For this review, take the finished solid that the model builds, in its own axes (mm). Face numbers are marked on the shaded views. A direction names the side the tool comes from. Coordinates: 2 decimals unless noted, no trailing zeros. Order: outer loops, then holes, each group sorted by start corner. A loop starts at its lowest first (then second) coordinate and runs counter-clockwise, first axis right, second up. Notation, with made-up numbers: M -34.5,36.5 L 3.5,36.5 A13 cw 3.5,44.5 Z; hole C 26.25,-34 d1. An arc over 180 degrees is marked long. Use CSV: the item, a comma, the result in double quotes.
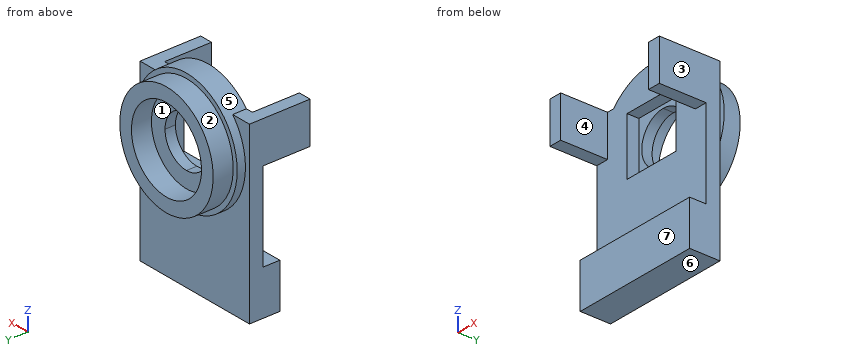
```python
from build123d import *

# Parameters (mm, degrees)
SKETCH2_W           = 8.34
SKETCH2_H           = 8.34
BOSS_EXTRUDE2_DEPTH = 1.5
CUT_EXTRUDE1_DEPTH  = 1.5
BOSS_EXTRUDE4_DEPTH = 3.2
SKETCH6_R           = 8.685
SKETCH6_W           = 11.34
SKETCH6_H           = 11.34
BOSS_EXTRUDE5_DEPTH = 3.2
SKETCH8_R           = 8
SKETCH8_R_2         = 6
BOSS_EXTRUDE6_DEPTH = 2.9
BOSS_EXTRUDE7_START = -2
BOSS_EXTRUDE7_DEPTH = 2
SKETCH11_W          = 18.74
SKETCH11_H          = 6.5
BOSS_EXTRUDE8_DEPTH = 2.4
SKETCH12_W          = 1.85
SKETCH12_H          = 6
BOSS_EXTRUDE9_DEPTH = 6.8


with BuildPart() as part:
    # Sketch2 → Boss-Extrude2 (new body)
    with BuildSketch(Plane(origin=(0, 0, 0), x_dir=(1, 0, 0), z_dir=(0, 1, 0))):
        with Locations((2.034857004, -1.978756257)):
            Rectangle(SKETCH2_W, SKETCH2_H)
    extrude(amount=BOSS_EXTRUDE2_DEPTH)

    # Sketch3 → Cut-Extrude1 (cut)
    with BuildSketch(Plane(origin=(0, 1.5, 0), x_dir=(1, 0, 0), z_dir=(0, 1, 0))):
        with BuildLine():
            ThreePointArc((5.704857004, -1.978756257), (4.629938891, 0.61632563), (2.034857004, 1.691243743))
            Line((2.034857004, 1.691243743), (2.034857004, -5.648756257))
            ThreePointArc((2.034857004, -5.648756257), (4.629938891, -4.573838143), (5.704857004, -1.978756257))
        make_face()
        with BuildLine():
            Line((2.034857004, -5.648756257), (2.034857004, 1.691243743))
            ThreePointArc((2.034857004, 1.691243743), (-1.635142996, -1.978756257), (2.034857004, -5.648756257))
        make_face()
    extrude(amount=-CUT_EXTRUDE1_DEPTH, mode=Mode.SUBTRACT)

    # Sketch5 → Boss-Extrude4 (add)
    with BuildSketch(Plane(origin=(0, 1.5, 0), x_dir=(1, 0, 0), z_dir=(0, 1, 0))):
        Polygon((-2.135142996, -6.148756257), (-2.135142996, 2.191243743), (-3.635142996, 2.191243743), (-3.635142996, -7.648756257), (6.204857004, -7.648756257), (6.204857004, -6.148756257), align=None)
        Polygon((7.704857004, 3.691243743), (7.704857004, -7.648756257), (6.204857004, -7.648756257), (6.204857004, -6.148756257), (6.204857004, 2.191243743), (-2.135142996, 2.191243743), (-3.635142996, 2.191243743), (-3.635142996, 3.691243743), align=None)
    extrude(amount=-BOSS_EXTRUDE4_DEPTH)

    # Sketch6 → Boss-Extrude5 (add)
    with BuildSketch(Plane(origin=(0, 1.5, 0), x_dir=(1, 0, 0), z_dir=(0, 1, 0))):
        with Locations(Location((2.034857004, -1.978756257, 0), (0, 0, 270))):
            Circle(SKETCH6_R)
        with Locations((2.034857004, -1.978756257)):
            Rectangle(SKETCH6_W, SKETCH6_H, mode=Mode.SUBTRACT)
    extrude(amount=-BOSS_EXTRUDE5_DEPTH)

    # Sketch8 → Boss-Extrude6 (add)
    with BuildSketch(Plane(origin=(0, 1.5, 0), x_dir=(1, 0, 0), z_dir=(0, 1, 0))):
        with Locations(Location((2.034857004, -1.978756257, 0), (0, 0, 90))):
            Circle(SKETCH8_R)
        with Locations(Location((2.034857004, -1.978756257, 0), (0, 0, 270))):
            Circle(SKETCH8_R_2, mode=Mode.SUBTRACT)
    extrude(amount=BOSS_EXTRUDE6_DEPTH)

    # Sketch10 → Boss-Extrude7 (add)
    with BuildSketch(Plane.XZ.offset(1.7).offset(BOSS_EXTRUDE7_START)):
        with BuildLine():
            Line((6.204857004, -17.591243743), (6.204857004, -5.639663855))
            ThreePointArc((6.204857004, -5.639663855), (-4.10636539, -4.162466138), (-5.583563108, 6.148756257))
            Line((-5.583563108, 6.148756257), (-7.335142996, 6.148756257))
            Line((-7.335142996, 6.148756257), (-7.335142996, -17.591243743))
            Line((-7.335142996, -17.591243743), (6.204857004, -17.591243743))
        make_face()
        with BuildLine():
            Line((-7.335142996, 6.148756257), (-5.583563108, 6.148756257))
            ThreePointArc((-5.583563108, 6.148756257), (-5.065192067, 6.980608732), (-4.456392875, 7.748756257))
            Line((-4.456392875, 7.748756257), (-7.335142996, 7.748756257))
            Line((-7.335142996, 7.748756257), (-7.335142996, 6.148756257))
        make_face()
        with BuildLine():
            ThreePointArc((8.526106884, 7.748756257), (9.134906076, 6.980608732), (9.653277116, 6.148756257))
            Line((9.653277116, 6.148756257), (11.404857004, 6.148756257))
            Line((11.404857004, 6.148756257), (11.404857004, 7.748756257))
            Line((11.404857004, 7.748756257), (8.526106884, 7.748756257))
        make_face()
        with BuildLine():
            ThreePointArc((10.719857004, 1.978756257), (9.506325233, -2.449153804), (6.204857004, -5.639663855))
            Line((6.204857004, -5.639663855), (6.204857004, -17.591243743))
            Line((6.204857004, -17.591243743), (11.404857004, -17.591243743))
            Line((11.404857004, -17.591243743), (11.404857004, 6.148756257))
            Line((11.404857004, 6.148756257), (9.653277116, 6.148756257))
            ThreePointArc((9.653277116, 6.148756257), (10.448988084, 4.130876877), (10.719857004, 1.978756257))
        make_face()
    extrude(amount=BOSS_EXTRUDE7_DEPTH)

    # Sketch11 → Boss-Extrude8 (add)
    with BuildSketch(Plane.XZ.offset(1.7)):
        with Locations((2.034857004, -14.341243743)):
            Rectangle(SKETCH11_W, SKETCH11_H)
    extrude(amount=BOSS_EXTRUDE8_DEPTH)

    # Sketch12 → Boss-Extrude9 (add)
    with BuildSketch(Plane.XZ.offset(1.7)):
        with Locations((-6.410142996, 4.748756257)):
            Rectangle(SKETCH12_W, SKETCH12_H)
        with Locations((10.479857004, 4.748756257)):
            Rectangle(SKETCH12_W, SKETCH12_H)
    extrude(amount=BOSS_EXTRUDE9_DEPTH)


solid = part.part
```
Item 1: Add section C-C on y = -0.75. State the section outline as (x, z) points (3 decimals).
Solutions:
outline,"M -7.335,-17.591 L 11.405,-17.591 L 11.405,7.749 L 8.526,7.749 A8.685 ccw -4.456,7.749 L -7.335,7.749 Z; hole M -2.135,-2.191 L 6.205,-2.191 L 6.205,6.149 L -2.135,6.149 Z"
Item 2: To check wall thickness, follow line 1 along X through (y, z) = (-4, 5.5); line 2 along Y through (x, z) = (-0.25, 7); line 3 along Y through (x, z) = (-0.75, -10.25). State the ranges of each line that lie inside material, in increasing order. Write a range as [from, to].
Solutions:
line 1,"[-7.34, -5.49], [9.55, 11.4]"
line 2,"[-1.7, 1.5]"
line 3,"[-1.7, 0.3]"
Item 3: Add section B-B on z = 0. State the section outline as (x, y) points, and give its area (3 significant figures).
Solutions:
outline,"M -7.34,-1.7 L -2.14,-1.7 L -2.14,0 L -1.06,0 L -1.06,1.5 L -3.63,1.5 L -3.63,4.4 L -5.72,4.4 L -5.72,1.5 L -6.42,1.5 L -6.42,0.3 L -7.34,0.3 Z; M 5.13,0 L 6.2,0 L 6.2,-1.7 L 11.4,-1.7 L 11.4,0.3 L 10.49,0.3 L 10.49,1.5 L 9.79,1.5 L 9.79,4.4 L 7.7,4.4 L 7.7,1.5 L 5.13,1.5 Z"
area,"46.4 mm^2"
Item 4: For the marked faces 4, 5, 6 and 7, list the 3-axis set-ups (+Z, -Z, +X, -X, +Y, -Y) from which the entire face can be reached by the end or side of a thin tool; tool diameter is ignored.
Solutions:
face 4,"+Z, -Y"
face 5,"+Y"
face 6,"-Z, +X, -X, +Y, -Y"
face 7,"-Z, +X, -X, -Y"
Item 5: Add section A-A on y = -7. State the section outline as (x, z) points.
Solutions:
outline,"M -7.34,1.75 L -5.49,1.75 L -5.49,7.75 L -7.34,7.75 Z; M 9.55,1.75 L 11.4,1.75 L 11.4,7.75 L 9.55,7.75 Z"
Item 6: Clearance check with flat-ended pins moving along their axes: pin 1 Ø2 at (x, y) = (-6.5, -6.5) entering from -Z; pin 2 Ø6 at (x, z) = (1.5, -8.5) entering from -Y; pin 3 Ø1.4 at (x, y) = (3.5, -1) entering from +Z. State where each tip first meets the part, or that it passes through.
Solutions:
pin 1,"z = 1.75"
pin 2,"y = -4.1"
pin 3,"z = 10.63"
Item 7: Draft analysis for pull direction Z (two halves, no side actions). For the marked faces 1, 2 and 3, state which applies: released by +Z, released by -Z, zero draft, split by the parting line, or undercut.
Solutions:
face 1,"undercut"
face 2,"split by the parting line"
face 3,"zero draft"
Item 8: Add section D-D on x = 4. State the section outline as (y, z) points.
Solutions:
outline,"M -4.1,-17.59 L 0.3,-17.59 L 0.3,-6.48 L 1.5,-6.48 L 1.5,-5.78 L 4.4,-5.78 L 4.4,-3.69 L 1.5,-3.69 L 1.5,-1.12 L 0,-1.12 L 0,-2.19 L -1.7,-2.19 L -1.7,-11.09 L -4.1,-11.09 Z; M -1.7,6.15 L 0,6.15 L 0,5.08 L 1.5,5.08 L 1.5,7.65 L 4.4,7.65 L 4.4,9.73 L 1.5,9.73 L 1.5,10.44 L -1.7,10.44 Z"
